from build123d import *

# Parameters (mm, degrees)
SKETCH1_R                = 1.5
BOSS_EXTRUDE1_DEPTH      = 116
SKETCH4_R                = 3
BOSS_EXTRUDE4_DEPTH      = 1
SKETCH7_R                = 1.5
REVOLVE1_ANGLE           = 80
BOSS_EXTRUDE5_DEPTH      = 4.5
BOSS_EXTRUDE5_DEPTH_BACK = 4.5
SKETCH8_R                = 1.5


with BuildPart() as part:
    # Sketch1 → Boss-Extrude1 (new body)
    with BuildSketch(Plane(origin=(0, 0, 0), x_dir=(1, 0, 0), z_dir=(0, 1, 0))):
        with Locations(Location((0, 0, 0), (0, 0, 90))):
            Circle(SKETCH1_R)
    extrude(amount=BOSS_EXTRUDE1_DEPTH)

    # Sketch4 → Boss-Extrude4 (add)
    with BuildSketch(Plane.XZ):
        with Locations(Location((0, 0, 0), (0, 0, 270))):
            Circle(SKETCH4_R)
    extrude(amount=BOSS_EXTRUDE4_DEPTH)

    # Sketch7 → Revolve1 (revolve)
    with BuildSketch(Plane(origin=(0, 116, 0), x_dir=(1, 0, 0), z_dir=(0, 1, 0))):
        with Locations(Location((0, 0, 0), (0, 0, 270))):
            Circle(SKETCH7_R)
    revolve(axis=Axis((-42.510122648, 116, -33.5), (-1, 0, 0)), revolution_arc=REVOLVE1_ANGLE)

    # Sketch8 → Boss-Extrude5 (add, two sides: drawn at the far end of the back side and taken through both)
    with BuildSketch(Plane(origin=(0, 0, 0), x_dir=(0, 0, -1), z_dir=(1, 0, 0)).offset(-BOSS_EXTRUDE5_DEPTH_BACK)):
        with Locations((27.682786048, 148.991059726)):
            Circle(SKETCH8_R)
    extrude(amount=BOSS_EXTRUDE5_DEPTH + BOSS_EXTRUDE5_DEPTH_BACK)


solid = part.part
Source: CAD feature listing. Evaluate the final solid. Frame: model axes, mm. A direction names the side the tool comes from. Coordinates: 2 decimals unless noted, no trailing zeros. Loops run counter-clockwise (first coordinate to the right, second up) from the corner with the lowest first, then second, coordinate; pieces in that order, holes last. Notation, with made-up numbers: (-25, 46) -> (5, 46) arc R15 cw to (5, 61) -> close; hole circle Ø5 at (35.5, 27.5). An arc over 180 degrees is marked (long way). Answer in a Markdown table with one row per item. Add a question column.
Q1. Reachability of faces 5 (the face through (-1.3, 0, -1.3)), 6 (the face through (0.9, -0.49, -2.86)), 7 (the face through (4.5, 149, -28)) from +Z, -Z, +X, -X, +Y, -Y: full face, straight path, thin tool, end or side. Return the list, or none.
Q2. Ray query, line 1 along Z through (x, y) = (0.25, 55.5); line 2 along Z through (x, y) = (-1.25, 47); line 3 along Y through (x, z) = (-0.5, -8). Return the intervals inside material, ascending.
Q3. Pull-direction query (Y, two-part tool) for faces 1 (the face through (-4.5, 149, -28)), 2 (the face through (0, -1, 0)), 3 (the face through (-0.063, 149.442, -29.114)), 4 (the face through (-0.45, 57.19, -1.43)); classes: pulls with the +Y half, pulls with the -Y half, needs draft (parallel to the pull), parting line crosses it, or undercut.
Q4. Section A-A on y = 91. Return the cut outline in (x, z), and give its area (3 significant figures).
Q5. Contact query for flat-ended pins moving along their axis: pin 1 Ø5 at (x, z) = (-2.5, -13) entering from -Y; pin 2 Ø4 at (x, z) = (-2.5, -17) entering from +Y; pin 3 Ø5 at (x, z) = (1, -15) entering from +Y. Output: stop coordinate, or through.
Computed values:
| question | item | result |
|---|---|---|
| 1 | face 5 | none |
| 1 | face 6 | -Y |
| 1 | face 7 | +Z, -Z, +X, +Y, -Y |
| 2 | line 1 | z = -1.48 to 1.48 |
| 2 | line 2 | z = -0.83 to 0.83 |
| 2 | line 3 | y = 135.47 to 139.85 |
| 3 | face 1 | needs draft |
| 3 | face 2 | pulls with the -Y half |
| 3 | face 3 | parting line crosses it |
| 3 | face 4 | undercut |
| 4 | outline | circle Ø3 at (0, 0) |
| 4 | area | 7.07 mm^2 |
| 5 | pin 1 | stops at y = 139.24 |
| 5 | pin 2 | stops at y = 147.15 |
| 5 | pin 3 | stops at y = 147.05 |
